Here's how the part is built. I have some questions about the finished solid (model axes, mm). Face numbers are marked on the shaded views. A direction names the side the tool comes from. Coordinates: 2 decimals unless noted, no trailing zeros. Write each loop counter-clockwise with the first axis right and the second up, starting at its lowest first coordinate (ties: lowest second). Pieces come first, ordered by that corner, then holes. Notation, with made-up numbers: (-17.75, 48.25) - (23.25, 48.25) arc R22 ccw to (23.25, 62.25) - close; hole circle Ø4 at (61.25, -35.5). An arc over 180 degrees is marked (long way). Answer in a Markdown table with one row per item. Add a question column.
Item 1: Imagine slicing it at C-C (y = 88). Please give me the cut outline in (x, z).
Item 2: We'd pull the mould along X, two halves only. Please class the marked faces 1, 2 and 3: +X half, -X half, draft (parallel to the pull), parting line (faces both ways), or undercut.
Item 3: Which directions (+Z, -Z, +X, -X, +Y, -Y) give clear straight access to the entire face, cutting with the end or side of a thin tool? Please do the marked faces 4 and 5.
Item 4: Imagine slicing it at B-B (z = 85). Please give me the cut outline in (x, y), plus the area to 3 significant figures.
Item 5: Imagine slicing it at A-A (y = 158.79). Please give me the cut outline in (x, z).
Item 6: If I drill on probe 1 along Y at (x, z) = (12.71, 132.6); probe 2 along Z at (x, y) = (-3.5, -5.05); probe 3 along X at (y, z) = (388, 132.7), over which ranges is the centre line in solid material (lowest first)? Write a range as from..to.
Item 7: Imagine slicing it at D-D (z = 115.5). Please give me the cut outline in (x, y), plus the area to 3 significant figures.
Item 8: I'm going to push flat-ended pins straight in: pin 1 (4 mm diameter, centred on x = 21, z = 71.5, fed in from -Y); pin 2 (24 mm diameter, centred on x = 12.71, y = 158.79, fed in from -Z); pin 3 (16 mm diameter, centred on x = -9.5, z = 84.5, fed in from -Y); pin 4 (4 mm diameter, centred on x = 0, y = 388, fed in from -Z). Where does each tip first touch, or does it pass through?
from build123d import *

# Parameters (mm, degrees)
F1_DEPTH      = 394
F2_W          = 65.42
F2_H          = 133.21
F3_DEPTH      = 1.21
F4_R          = 27.6
F5_DEPTH      = 395.211
F6_R          = 12.6
F7_DEPTH      = 395.211
F7_DEPTH_BACK = 628
F8_R          = 20
F8_R_2        = 12.6
F9_DEPTH      = 6.4
F11_R         = 7.5
F12_DEPTH     = 133.211
F13_R         = 3.25
F14_DEPTH     = 25
F10_R         = 16
F15_DEPTH     = 4
F16_R         = 3.1
F17_DEPTH     = 395.211


# Not quite as in the source:
# - an extrude ends at something that could not be found from the text; its depth is read off the source's solid


with BuildPart() as f1:
    # F0 (on Front) → F1 (new body)
    with BuildSketch(Plane.XZ):
        Polygon((-31.5, 132), (0, 132), (31.5, 132), (31.5, 0), (32.71, 0), (32.71, 133.21), (0, 133.21), (-32.71, 133.21), (-32.71, 0), (-31.5, 0), align=None)
    extrude(amount=-F1_DEPTH)

    # F2 (on face) → F3 (join)
    with BuildSketch(Plane.XZ):
        with Locations((0, 66.605)):
            Rectangle(F2_W, F2_H)
    extrude(amount=F3_DEPTH)

    # F4 (on face) → F5 (cut, through all)
    with BuildSketch(Plane.XZ.offset(1.21)):
        with Locations((0, 32)):
            Circle(F4_R)
    extrude(amount=-F5_DEPTH, mode=Mode.SUBTRACT)

    # F6 (on face) → F7 (cut, two sides)
    with BuildSketch(Plane.XZ.offset(1.21)) as f7_sk:
        with Locations((-3.5, 85)):
            Circle(F6_R)
    extrude(amount=-F7_DEPTH, mode=Mode.SUBTRACT)
    extrude(f7_sk.sketch, amount=F7_DEPTH_BACK, mode=Mode.SUBTRACT)

    # F8 (on face) → F9 (join)
    with BuildSketch(Plane.XZ.offset(1.21)):
        with Locations((-3.5, 85)):
            Circle(F8_R)
        with Locations((-3.5, 85)):
            Circle(F8_R_2, mode=Mode.SUBTRACT)
    extrude(amount=F9_DEPTH)

    # F11 (on face) → F12 (cut, through all)
    with BuildSketch(Plane.XY.offset(133.21)):
        with Locations((12.71, 68.79)):
            Circle(F11_R)
        with Locations((12.71, 113.79)):
            Circle(F11_R)
        with Locations((12.71, 158.79)):
            Circle(F11_R)
    extrude(amount=-F12_DEPTH, mode=Mode.SUBTRACT)

    # F13 (on face) → F14 (cut)
    with BuildSketch(Plane.XY.offset(133.21)):
        with Locations((0, 388)):
            Circle(F13_R)
    extrude(amount=-F14_DEPTH, mode=Mode.SUBTRACT)

    # F10 (on face) → F15 (cut)
    with BuildSketch(Plane.XZ.offset(7.61)):
        with Locations((-3.5, 85)):
            Circle(F10_R)
    extrude(amount=-F15_DEPTH, mode=Mode.SUBTRACT)

    # F16 (on face) → F17 (cut, through all)
    with BuildSketch(Plane.XZ.offset(1.21)):
        with Locations((20, 57)):
            Circle(F16_R)
        with Locations((-20, 57)):
            Circle(F16_R)
        with Locations((-20, 7)):
            Circle(F16_R)
        with Locations((20, 7)):
            Circle(F16_R)
    extrude(amount=-F17_DEPTH, mode=Mode.SUBTRACT)


solid = f1.part
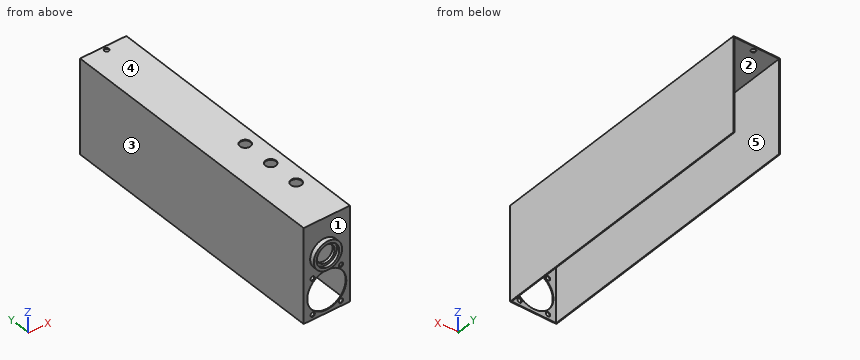
Here are the results:
| question | item | result |
|---|---|---|
| 1 | outline | (-32.71, 0) - (-31.5, 0) - (-31.5, 132) - (31.5, 132) - (31.5, 0) - (32.71, 0) - (32.71, 133.21) - (-32.71, 133.21) - close |
| 2 | face 1 | draft |
| 2 | face 2 | undercut |
| 2 | face 3 | -X half |
| 3 | face 4 | +Z, +X, -X, +Y, -Y |
| 3 | face 5 | -Z, +Y |
| 4 | outline | (-32.71, -1.21) - (-23.5, -1.21) - (-23.5, -7.61) - (-19.5, -7.61) - (-19.5, -3.61) - (-16.1, -3.61) - (-16.1, 0) - (-31.5, 0) - (-31.5, 394) - (-32.71, 394) - close; (9.1, -3.61) - (12.5, -3.61) - (12.5, -7.61) - (16.5, -7.61) - (16.5, -1.21) - (32.71, -1.21) - (32.71, 394) - (31.5, 394) - (31.5, 0) - (9.1, 0) - close |
| 4 | area | 1,070 mm2 |
| 5 | outline | (-32.71, 0) - (-31.5, 0) - (-31.5, 132) - (5.21, 132) - (5.21, 133.21) - (-32.71, 133.21) - close; (20.21, 132) - (31.5, 132) - (31.5, 0) - (32.71, 0) - (32.71, 133.21) - (20.21, 133.21) - close |
| 6 | probe 1 | y = -1.21..61.29, 76.29..106.29, 121.29..151.29, 166.29..394 |
| 6 | probe 2 | z = 65..69, 101..105 |
| 6 | probe 3 | x = -32.71..-3.25, 3.25..32.71 |
| 7 | outline | (-32.71, -1.21) - (32.71, -1.21) - (32.71, 394) - (31.5, 394) - (31.5, 0) - (-31.5, 0) - (-31.5, 394) - (-32.71, 394) - close |
| 7 | area | 1,030 mm2 |
| 8 | pin 1 | stops at y = -1.21 |
| 8 | pin 2 | stops at z = 132 |
| 8 | pin 3 | stops at y = -3.61 |
| 8 | pin 4 | passes through |
